from build123d import *

# Parameters (mm, degrees)
ACRYLIC_SHEET_W     = 482.6
ACRYLIC_SHEET_H     = 127
BOSS_EXTRUDE1_DEPTH = 6.35
SKETCH2_W           = 482.6
SKETCH2_H           = 19.05
BOSS_EXTRUDE2_DEPTH = 88.9


with BuildPart() as part:
    # Acrylic Sheet → Boss-Extrude1 (new body)
    with BuildSketch(Plane(origin=(0, 0, 0), x_dir=(1, 0, 0), z_dir=(0, 1, 0))):
        with Locations((241.3, 63.5)):
            Rectangle(ACRYLIC_SHEET_W, ACRYLIC_SHEET_H)
    extrude(amount=BOSS_EXTRUDE1_DEPTH)

    # Sketch2 → Boss-Extrude2 (add)
    with BuildSketch(Plane(origin=(0, 6.35, 0), x_dir=(1, 0, 0), z_dir=(0, 1, 0))):
        with Locations((241.3, 9.525)):
            Rectangle(SKETCH2_W, SKETCH2_H)
        with Locations((241.3, 117.475)):
            Rectangle(SKETCH2_W, SKETCH2_H)
    extrude(amount=BOSS_EXTRUDE2_DEPTH)


solid = part.part
Could you check a few things on this model? Use its own coordinates, in mm. A direction names the side the tool comes from. Round coordinates to 2 decimals unless told otherwise and drop trailing zeros. Loops run counter-clockwise (first coordinate to the right, second up) from the corner with the lowest first, then second, coordinate; pieces in that order, holes last. Notation, with made-up numbers: (79, 5.25) - (117, 5.25) arc R4 ccw to (117, 9.25) - close; hole circle Ø5 at (73, 16.5). An arc over 180 degrees is marked (long way). Write item = value, one per line.
1) If we mould it in two halves opening along Z, with no side actions, what happens to faces 1 (the flat face through (238, 6.35, -64)), 2 (the flat face through (238, 95.25, -118)), 3 (the flat face through (238, 47, -127))? For each: pulls with the +Z half, pulls with the -Z half, needs draft (parallel to the pull), parting line crosses it, or undercut.
Computed:
face_1 = undercut
face_2 = needs draft
face_3 = pulls with the -Z half
2) Imagine slicing it at B-B (x = 167). Please give me the cut outline in (y, z).
Computed:
outline = (0, -127) - (95.25, -127) - (95.25, -107.95) - (6.35, -107.95) - (6.35, -19.05) - (95.25, -19.05) - (95.25, 0) - (0, 0) - close
3) On a 3-axis mill with a long thin cutter (end or side, diameter ignored), from which of +Z, -Z, +X, -X, +Y, -Y can I reach the whole of each face in a straight line? I mean faces 4 (the flat face through (238, 50, -107.95)), 5 (the flat face through (482.6, 5, -54)). Say none if no direction works.
Computed:
face_4 = +X, -X, +Y
face_5 = +Z, -Z, +X, +Y, -Y
4) Imagine slicing it at A-A (y = 57). Please give me the cut outline in (x, z), and give its area (3 significant figures).
Computed:
outline = (0, -127) - (482.6, -127) - (482.6, -107.95) - (0, -107.95) - close; (0, -19.05) - (482.6, -19.05) - (482.6, 0) - (0, 0) - close
area = 18,400 mm2
5) I need wall thicknesses on line 1 along Z through (x, y) = (134, 13); line 2 along Y through (x, z) = (266, -93.5). Which ranges of each line are inside material? Lowest first, please. Write a range as from..to.
Computed:
line_1 = -127..-107.95, -19.05..0
line_2 = 0..6.35
6) I'm going to push a flat-ended pin straight in: P1, Ø10, axis at x = 74, z = -30, coming from the +Y side. Where does the tip first touch, or does it pass through?
Computed:
P1 = 6.35
7) Imagine slicing it at C-C (z = -64). Please give me the cut outline in (x, y).
Computed:
outline = (0, 0) - (482.6, 0) - (482.6, 6.35) - (0, 6.35) - close
